```python
from build123d import *

# Parameters (mm, degrees)
PAD008_DEPTH    = 100
SKETCH013_R     = 2
SKETCH013_W     = 1.5
SKETCH013_H     = 4
PAD_DEPTH       = 2
SKETCH005_W     = 6
SKETCH005_H     = 37
SKETCH005_H_2   = 35
POCKET013_DEPTH = 20
SKETCH009_W     = 8
SKETCH009_H     = 3.1
POCKET014_DEPTH = 20
SKETCH007_W     = 5
SKETCH007_H     = 37
POCKET015_DEPTH = 5
SKETCH021_R     = 18
POCKET018_DEPTH = 5


with BuildPart() as part:
    # Sketch004 → Pad008 (new body)
    with BuildSketch(Plane.YZ.offset(100)):
        Polygon((7, 12), (16, 12), (16, 6), (20, 6), (20, 16), (0, 16), (0, 6), (7, 6), align=None)
    extrude(amount=-PAD008_DEPTH)

    # Sketch013 → Pad (new body)
    with BuildSketch(Plane(origin=(100, 0, 6), x_dir=(0, 1, 0), z_dir=(0, 0, -1))):
        with Locations((3, -4)):
            Circle(SKETCH013_R)
        with Locations((3, -96)):
            Circle(SKETCH013_R)
        with Locations((17.75, -4)):
            Rectangle(SKETCH013_W, SKETCH013_H)
    extrude(amount=PAD_DEPTH)

    # Sketch005 → Pocket013 (cut)
    with BuildSketch(Plane(origin=(100, 0, 0), x_dir=(0, 0, -1), z_dir=(0, -1, 0))):
        with Locations((-9, -28.5)):
            Rectangle(SKETCH005_W, SKETCH005_H)
        with Locations((-9, -74)):
            Rectangle(SKETCH005_W, SKETCH005_H_2)
    extrude(amount=-POCKET013_DEPTH, mode=Mode.SUBTRACT)

    # Sketch009 → Pocket014 (cut)
    with BuildSketch(Plane(origin=(100, 0, 0), x_dir=(0, 0, -1), z_dir=(0, -1, 0))):
        with Locations((-17, -95.55)):
            Rectangle(SKETCH009_W, SKETCH009_H)
    extrude(amount=-POCKET014_DEPTH, mode=Mode.SUBTRACT)

    # Sketch007 → Pocket015 (cut)
    with BuildSketch(Plane(origin=(100, 0, 16), x_dir=(0, -1, 0), z_dir=(0, 0, 1))):
        with BuildLine():
            ThreePointArc((-20, -85.5), (-12.499999, -78), (-20, -70.5))
            Line((-20, -85.5), (-20, -70.5))
        make_face()
        with Locations((-17.5, -28.5)):
            Rectangle(SKETCH007_W, SKETCH007_H)
        with Locations((-2.5, -28.5)):
            Rectangle(SKETCH007_W, SKETCH007_H)
    extrude(amount=-POCKET015_DEPTH, mode=Mode.SUBTRACT)

    # Sketch021 → Pocket018 (cut)
    with BuildSketch(Plane(origin=(100, 0, 6), x_dir=(0, 1, 0), z_dir=(0, 0, -1))):
        with Locations((20, -78)):
            Circle(SKETCH021_R)
    extrude(amount=-POCKET018_DEPTH, mode=Mode.SUBTRACT)


solid = part.part
```
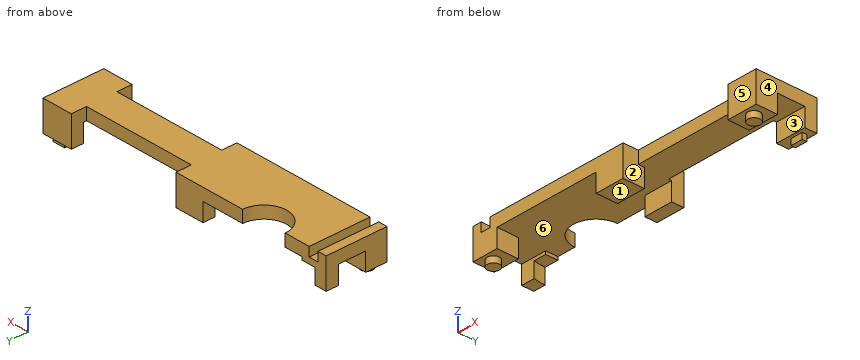
Source: CAD feature listing. Evaluate the final solid. Frame: model axes, mm. Face numbers are marked on the shaded views. A direction names the side the tool comes from. Round coordinates to 2 decimals unless told otherwise and drop trailing zeros. Loops run counter-clockwise (first coordinate to the right, second up) from the corner with the lowest first, then second, coordinate; pieces in that order, holes last.
(1) Section query A-A (z = 8). Output: boundary loops of the cut face in (x, y), and give its area (3 significant figures).
From the geometry:
outline: (0, 0) - (8.5, 0) - (8.5, 7) - (0, 7) - close; (0, 16) - (4.45, 16) arc R18 cw to (4, 20) - (0, 20) - close; (43.5, 0) - (53, 0) - (53, 7) - (43.5, 7) - close; (43.5, 16) - (53, 16) - (53, 20) - (43.5, 20) - close; (90, 0) - (100, 0) - (100, 7) - (90, 7) - close; (90, 16) - (100, 16) - (100, 20) - (90, 20) - close
area: 291 mm2
(2) Material intervals for probe 1 along X at (y, z) = (1.25, 10.5); probe 2 along X at (y, z) = (4, 15); probe 3 along X at (y, z) = (11, 15.75), sorted ascending.
From the geometry:
probe 1: x = 0 to 8.5, 43.5 to 53, 90 to 100
probe 2: x = 0 to 2.9, 6 to 53, 90 to 100
probe 3: x = 0 to 2.9, 6 to 100
(3) Section query D-D (x = 41.5). Output: boundary loops of the cut face in (y, z).
From the geometry:
outline: (0, 12) - (20, 12) - (20, 16) - (0, 16) - close
(4) Section query B-B (y = 3). Output: boundary loops of the cut face in (x, z).
From the geometry:
outline: (0, 6) - (2, 6) - (2, 4) - (6, 4) - (6, 6) - (8.5, 6) - (8.5, 12) - (43.5, 12) - (43.5, 6) - (53, 6) - (53, 16) - (6, 16) - (6, 13) - (2.9, 13) - (2.9, 16) - (0, 16) - close; (90, 6) - (94, 6) - (94, 4) - (98, 4) - (98, 6) - (100, 6) - (100, 16) - (90, 16) - close
(5) Section query C-C (x = 96). Output: boundary loops of the cut face in (y, z).
From the geometry:
outline: (0, 6) - (1, 6) - (1, 4) - (5, 4) - (5, 6) - (7, 6) - (7, 12) - (16, 12) - (16, 6) - (17, 6) - (17, 4) - (18.5, 4) - (18.5, 6) - (20, 6) - (20, 16) - (0, 16) - close
(6) Access query for the marked faces 1, 2 and 3. Directions: +Z, -Z, +X, -X, +Y, -Y. A direction counts if a zero-diameter tool reaches every point of the face in a straight line with its end or side. Return the directions, or none.
From the geometry:
face 1: -Z, +Y, -Y
face 2: -Z, -Y
face 3: -Z, +X, -X
(7) Contact query for flat-ended pins moving along their axis: pin 1 Ø2 at (x, y) = (59, 10.5) entering from -Z; pin 2 Ø2 at (x, y) = (49, 4.5) entering from -Z; pin 3 Ø1.2 at (y, z) = (17.5, 5) entering from +X. Output: stop coordinate, or through.
From the geometry:
pin 1: stops at z = 12
pin 2: stops at z = 6
pin 3: stops at x = 98
(8) Pull-direction query (X, two-part tool) for the marked faces 4, 5 and 6; classes: +X half, -X half, draft (parallel to the pull), parting line (faces both ways), or undercut.
From the geometry:
face 4: +X half
face 5: draft
face 6: undercut
